CAD build for the part. Positions are in the model's coordinates, mm. A direction names the side the tool comes from. Round coordinates to 2 decimals unless told otherwise and drop trailing zeros. Order: outer loops, then holes, each group sorted by start corner. A loop starts at its lowest first (then second) coordinate and runs counter-clockwise, first axis right, second up. Notation, with made-up numbers: M 30.5,-21 L 57.5,-21 A22 cw 57.5,-15 Z; hole C -31.5,33.25 d11. An arc over 180 degrees is marked long. Put each result on its own line as item: value.
```python
from build123d import *

# Parameters (mm, degrees)
F0_W      = 1524
F0_H      = 762
F1_DEPTH  = 25.4
F2_W      = 25.4
F2_H      = 304.8
F3_DEPTH  = 685.8
F5_W      = 25.4
F5_H      = 609.6
F4_W      = 25.4
F4_H      = 609.6
F6_DEPTH  = 25.4
F7_W      = 25.4
F7_H      = 203.2
F8_DEPTH  = 1473.2
F9_W      = 25.4
F9_H      = 762
F10_DEPTH = 76.2


with BuildPart() as f1:
    # F0 (on Top) → F1 (new body)
    with BuildSketch(Plane.XY):
        Rectangle(F0_W, F0_H)
    extrude(amount=-F1_DEPTH)

    # F2 (on face) → F3 (join)
    with BuildSketch(Plane(origin=(0, 0, -25.4), x_dir=(1, 0, 0), z_dir=(0, 0, -1))):
        with Locations((749.3, -152.4)):
            Rectangle(F2_W, F2_H)
        with Locations((-749.3, -152.4)):
            Rectangle(F2_W, F2_H)
    extrude(amount=F3_DEPTH)

    # F5 (on face) + F4 (on face) → F6 (join)
    with BuildSketch(Plane(origin=(0, 0, -711.2), x_dir=(1, 0, 0), z_dir=(0, 0, -1))):
        with Locations((-749.3, 0)):
            Rectangle(F5_W, F5_H)
    with BuildSketch(Plane(origin=(0, 0, -711.2), x_dir=(1, 0, 0), z_dir=(0, 0, -1))):
        with Locations((749.3, 0)):
            Rectangle(F4_W, F4_H)
    extrude(amount=F6_DEPTH)

    # F7 (on face) → F8 (join, through all)
    with BuildSketch(Plane.YZ.offset(-736.6)):
        with Locations((292.1, -127)):
            Rectangle(F7_W, F7_H)
    extrude(amount=F8_DEPTH)

    # F9 (on face) → F10 (join)
    with BuildSketch(Plane.XY):
        with Locations((749.3, 0)):
            Rectangle(F9_W, F9_H)
        with Locations((-749.3, 0)):
            Rectangle(F9_W, F9_H)
    extrude(amount=F10_DEPTH)


solid = f1.part
```
Item 1: Pin check, flat tips, straight feed: P1, Ø3, axis at x = -533, y = -3.5, coming from the -Z side; P2, Ø1.5, axis at x = 74.5, y = 283, coming from the +Z side; P3, Ø7.5, axis at x = -750.5, z = -457, coming from the -Y side. Stop position of each tip, or through.
Answers below:
P1: z = -25.4
P2: z = 0
P3: y = 0
Item 2: Tool access for faces 1 (the flat face through (736.6, -5, 38)), 2 (the flat face through (736.6, 140, -376)), 3 (the flat face through (-60, 304.8, -198)): list every direction of +Z, -Z, +X, -X, +Y, -Y with a clear straight run to the whole face (end or side of a thin tool).
Answers below:
face 1: +Z, +Y, -Y
face 2: -Z, -Y
face 3: -Z, +X, -X, +Y
Item 3: Band-saw the part on D-D on z = -75.5. Give the cut face in (x, y).
Answers below:
outline: M -762,0 L -736.6,0 L -736.6,279.4 L 736.6,279.4 L 736.6,0 L 762,0 L 762,304.8 L -762,304.8 Z
Item 4: Band-saw the part on B-B on z = -256.5. Give the cut face in (x, y).
Answers below:
outline: M -762,0 L -736.6,0 L -736.6,304.8 L -762,304.8 Z; M 736.6,0 L 762,0 L 762,304.8 L 736.6,304.8 Z
Item 5: Probe line 1 along X through (y, z) = (222, 2.5); line 2 along Z through (x, y) = (575.5, -276.5); line 3 along Y through (x, z) = (235, -209). List the from-to ranges inside material, lowest first. Write a range as [from, to].
Answers below:
line 1: [-762, -736.6], [736.6, 762]
line 2: [-25.4, 0]
line 3: [279.4, 304.8]
Item 6: Band-saw the part on C-C on y = 18. Give the cut face in (x, z).
Answers below:
outline: M -762,-736.6 L -736.6,-736.6 L -736.6,-25.4 L 736.6,-25.4 L 736.6,-736.6 L 762,-736.6 L 762,76.2 L 736.6,76.2 L 736.6,0 L -736.6,0 L -736.6,76.2 L -762,76.2 Z
Item 7: Band-saw the part on A-A on y = -67. Give the cut face in (x, z).
Answers below:
outline: M -762,-736.6 L -736.6,-736.6 L -736.6,-711.2 L -762,-711.2 Z; M -762,-25.4 L 762,-25.4 L 762,76.2 L 736.6,76.2 L 736.6,0 L -736.6,0 L -736.6,76.2 L -762,76.2 Z; M 736.6,-736.6 L 762,-736.6 L 762,-711.2 L 736.6,-711.2 Z
Item 8: Mould opens along X. For faces 4 (the flat face through (-60, 381, -5)), 5 (the flat face through (-736.6, 140, -376)), 6 (the flat face through (762, 79, -246)) say: pulls with the +X half, pulls with the -X half, needs draft (parallel to the pull), parting line crosses it, or undercut.
Answers below:
face 4: needs draft
face 5: undercut
face 6: pulls with the +X half
